from build123d import *

# Parameters (mm, degrees)
F0_W      = 731.52
F0_H      = 731.52
F1_DEPTH  = 45.72
F3_W      = 734.7105741501
F3_H      = 731.8749427795
F4_DEPTH  = 45.72
F5_W      = 60.96
F5_H      = 60.96
F6_W      = 60.96
F6_H      = 60.96
F12_R     = 27.8235207136
F13_DEPTH = 6.096
F14_R     = 22.7734806104
F15_DEPTH = 60.96
F16_W     = 256.0497522354
F16_H     = 156.4687490463
F16_R     = 22.7734806104
F17_DEPTH = 24.384


with BuildPart() as f1:
    # F0 (on Top) → F1 (new body)
    with BuildSketch(Plane.XY):
        with Locations((365.76, -365.76)):
            Rectangle(F0_W, F0_H)
    extrude(amount=F1_DEPTH)

    # F14 (on face) → F15 (join)
    with BuildSketch(Plane(origin=(0, 0, 0), x_dir=(1, 0, 0), z_dir=(0, 0, -1))):
        with Locations((333.9223861694, 398.3253240585)):
            Circle(F14_R)
    extrude(amount=F15_DEPTH)



with BuildPart() as f4:
    # F3 (on offset) → F4 (new body)
    with BuildSketch(Plane.XY.offset(-1828.8)):
        with Locations((367.355287075, -365.9374713898)):
            Rectangle(F3_W, F3_H)
    extrude(amount=F4_DEPTH)

    # F12 (on face) → F13 (cut)
    with BuildSketch(Plane.XY.offset(-1783.08)):
        with Locations((333.7072134018, -305.7377934456)):
            Circle(F12_R)
    extrude(amount=-F13_DEPTH, mode=Mode.SUBTRACT)


with BuildPart() as f7:
    # F5 (on face) → F7 section 0
    with BuildSketch(Plane(origin=(0, 0, 0), x_dir=(1, 0, 0), z_dir=(0, 0, -1))):
        with Locations((701.04, 701.04)):
            Rectangle(F5_W, F5_H)
    # F6 (on face) → F7 section 1
    with BuildSketch(Plane.XY.offset(-1783.08)):
        with Locations((704.2305741501, -701.3949427795)):
            Rectangle(F6_W, F6_H)
    loft()


with BuildPart() as f8_1:
    # F8: instance of F7
    add(f7.part.mirror(Plane.YZ))


with BuildPart() as f11_1:
    # F11: instance of F7
    add(f7.part.mirror(Plane.YZ.offset(366.6744)))


with BuildPart() as f1_1:
    add(f1.part)

    add(f4.part)  # F17 merges F4

    add(f7.part)  # F17 merges F7

    add(f11_1.part)  # F17 merges F11_1
    # F16 (on face) → F17 (join)
    with BuildSketch(Plane(origin=(0, 0, -60.96), x_dir=(1, 0, 0), z_dir=(0, 0, -1))):
        with Locations((333.9223861694, 398.3253240585)):
            Rectangle(F16_W, F16_H)
        with Locations((333.9223861694, 398.3253240585)):
            Circle(F16_R, mode=Mode.SUBTRACT)
        with Locations((333.9223861694, 398.3253240585)):
            Circle(F16_R)
    extrude(amount=F17_DEPTH)


solid = f1_1.part
The model under review builds one solid part; all positions refer to its coordinate system, in mm. A direction names the side the tool comes from. Coordinates: 2 decimals unless noted, no trailing zeros. Order: outer loops, then holes, each group sorted by start corner. A loop starts at its lowest first (then second) coordinate and runs counter-clockwise, first axis right, second up. Notation, with made-up numbers: (-34.75, 65) -> (-1.75, 65) arc R24 cw to (-1.75, 76) -> close; hole circle Ø11 at (-15, -19.75). An arc over 180 degrees is marked (long way). Answer in a Markdown table with one row per item.
(1) Consider section C-C (x = 617). Write out the cut boundary in (y, z), plus the area to 3 significant figures.
Answers:
| item | result |
|---|---|
| outline | (-731.87, -1828.8) -> (0, -1828.8) -> (0, -1783.08) -> (-731.87, -1783.08) -> close; (-731.52, 0) -> (0, 0) -> (0, 45.72) -> (-731.52, 45.72) -> close |
| area | 66,900 mm² |
(2) Wall thickness on line 1 along Z through (x, y) = (263, -361); line 2 along Z through (x, y) = (147, -485); line 3 along Y through (x, z) = (48.5, -412.5): over which ranges is each line inside the solid? List them lowest first.
Answers:
| item | result |
|---|---|
| line 1 | -1828.8 to -1783.08, -85.34 to -60.96, 0 to 45.72 |
| line 2 | -1828.8 to -1783.08, 0 to 45.72 |
| line 3 | -731.6 to -670.64 |
(3) Consider section A-A (y = -156). Write out the cut boundary in (x, z), plus the area to 3 significant figures.
Answers:
| item | result |
|---|---|
| outline | (0, -1828.8) -> (734.71, -1828.8) -> (734.71, -1783.08) -> (0, -1783.08) -> close; (0, 0) -> (731.52, 0) -> (731.52, 45.72) -> (0, 45.72) -> close |
| area | 67,000 mm² |
(4) Machinability: for faces 4 (the flat face through (734.711, -371, -1806)), 5 (the flat face through (731.52, -371, 23)), 6 (the flat face through (362, 0, -1806)), 7 (the cylindrical face through (360.246, -297.38, -1786.085)), 8 (the flat face through (332, -399, -85.344)), which of the approach directions +Z, -Z, +X, -X, +Y, -Y give a long, thin tool a straight path to every point of the face, cutting with its end or side? Answer none if there is none.
Answers:
| item | result |
|---|---|
| face 4 | +Z, -Z, +X, +Y, -Y |
| face 5 | +Z, +X, +Y, -Y |
| face 6 | +Z, -Z, +X, -X, +Y |
| face 7 | none |
| face 8 | +X, -X, +Y, -Y |
(5) The part is to be moulded in two halves that separate along Z. For faces 1 (the flat face through (361, -399, -60.96)), 2 (the flat face through (362, -361, -1828.8)), 3 (the flat face through (0, -371, 23)), say which applies: +Z half, -Z half, draft (parallel to the pull), parting line (faces both ways), or undercut.
Answers:
| item | result |
|---|---|
| face 1 | undercut |
| face 2 | -Z half |
| face 3 | draft |
(6) Insertion check: pin 1 (1.1 mm diameter, centred on x = -1, y = -697, fed in from -Z); pin 2 (12 mm diameter, centred on x = 273.5, z = -68, fed in from -Y); pin 3 (23 mm diameter, centred on y = -284, z = -1799.5, fed in from -X). Each pin has a flat end and moves straight along its axis. Give the tip position at first contact, or say it passes through.
Answers:
| item | result |
|---|---|
| pin 1 | z = -1783.08 |
| pin 2 | y = -476.56 |
| pin 3 | x = 0 |
(7) Consider section B-B (x = 280). Write out the cut boundary in (y, z).
Answers:
| item | result |
|---|---|
| outline | (-731.87, -1828.8) -> (0, -1828.8) -> (0, -1783.08) -> (-731.87, -1783.08) -> close; (-731.52, 0) -> (0, 0) -> (0, 45.72) -> (-731.52, 45.72) -> close; (-476.56, -85.34) -> (-320.09, -85.34) -> (-320.09, -60.96) -> (-476.56, -60.96) -> close |
